Read the model definition and answer for the solid it produces. Units are mm, in the model's axes. A direction names the side the tool comes from. Give positions to 0.01 mm unless a question says otherwise; leave off trailing zeros. Order: outer loops, then holes, each group sorted by start corner. A loop starts at its lowest first (then second) coordinate and runs counter-clockwise, first axis right, second up.
```python
from build123d import *

# Parameters (mm, degrees)
SKETCH1_W           = 300
SKETCH1_H           = 125
BOSS_EXTRUDE2_DEPTH = 80
CUT_EXTRUDE2_DEPTH  = 135
SHELL2_T            = -2


with BuildPart() as part:
    # Sketch1 → Boss-Extrude2 (new body)
    with BuildSketch(Plane(origin=(0, 0, 0), x_dir=(1, 0, 0), z_dir=(0, 1, 0))):
        with Locations((-150, 62.5)):
            Rectangle(SKETCH1_W, SKETCH1_H)
    extrude(amount=BOSS_EXTRUDE2_DEPTH)

    # Sketch3 → Cut-Extrude2 (cut)
    with BuildSketch(Plane.XY):
        Polygon((0, 80), (-285, 80), (0, 40), align=None)
    extrude(amount=-CUT_EXTRUDE2_DEPTH, mode=Mode.SUBTRACT)

    # Shell2
    shell2_openings = [part.faces().sort_by_distance(p)[0] for p in [
        (-292.5, 80, -62.5),
        (-142.5, 60, -62.5),
        (0, 20, -62.5),
    ]]
    offset(amount=SHELL2_T, openings=shell2_openings, kind=Kind.INTERSECTION)


solid = part.part
```
1) A tool of negligible diameter and unlimited length cuts with its end or side. For faces 4 (the face through (-298, 40, -62)), 5 (the face through (-300, 39, -62)), from which of +Z, -Z, +X, -X, +Y, -Y can it reach the whole face along a straight path? Write none if from no direction.
Final values:
face 4: +X, +Y
face 5: +Z, -Z, -X, +Y, -Y
2) The part is cut by section C-C on x = -160. Determine the outline of the cut face in (y, z), and give its area (3 significant figures).
Final values:
outline: (0, -125) - (62.46, -125) - (62.46, -123) - (2, -123) - (2, -2) - (62.46, -2) - (62.46, 0) - (0, 0) - close
area: 492 mm2
3) The part is cut by section B-B on z = -24.5. Determine the outline of the cut face in (x, y).
Final values:
outline: (-300, 0) - (0, 0) - (0, 2) - (-298, 2) - (-298, 80) - (-300, 80) - close
4) Consider L1, parallel to Z at x = -258.5, y = 22.5; L2, parallel to Y at x = -140.5, z = -83; L3, parallel to X at y = 6, z = -77.5. Determine where each line is inside the solid, lowest interval first.
Final values:
L1: z = -125 to -123, -2 to 0
L2: y = 0 to 2
L3: x = -300 to -298
5) The part is cut by section A-A on y = 28. Determine the outline of the cut face in (x, z), and give its area (3 significant figures).
Final values:
outline: (-300, -125) - (0, -125) - (0, -123) - (-298, -123) - (-298, -2) - (0, -2) - (0, 0) - (-300, 0) - close
area: 1,440 mm2
6) For a pull along Z with two mould halves and no side action, classify faces 1 (the face through (-185, 31, -125)), 2 (the face through (-185, 31, 0)), 3 (the face through (-184, 32, -123)) as released by +Z, released by -Z, zero draft, split by the parting line, or undercut.
Final values:
face 1: released by -Z
face 2: released by +Z
face 3: undercut
7) Given pin 1 (3 mm diameter, centred on y = 64, z = -25, fed in from +X); pin 2 (12 mm diameter, centred on x = -269.5, z = -43.5, fed in from +Y), each flat-ended and moving along its own axis, determine where each tip first touches the part or whether it passes through.
Final values:
pin 1: stops at x = -298
pin 2: stops at y = 2
